Source: CAD feature listing. Evaluate the final solid. Frame: model axes, mm. A direction names the side the tool comes from. Coordinates: 2 decimals unless noted, no trailing zeros. Order: outer loops, then holes, each group sorted by start corner. A loop starts at its lowest first (then second) coordinate and runs counter-clockwise, first axis right, second up.
Item 1: Section A-A on x = 0. Return the cut outline in (y, z).
Item 2: Section B-B on z = -10.26. Return the cut outline in (x, y).
Item 3: Reachability of faces 5 (the flat face through (17, -6, -16)), 6 (the flat face through (-1, -6, -18)) from +Z, -Z, +X, -X, +Y, -Y: full face, straight path, thin tool, end or side. Return the list, or none.
Item 4: Section D-D on z = -2.75. Return the cut outline in (x, y).
Item 5: Contact query for flat-ended pins moving along their axis: P1, Ø4, axis at x = -23, y = -5.5, coming from the +Z side; P2, Ø8, axis at x = -25.5, z = -6.5, coming from the -Y side. Output: stop coordinate, or through.
Item 6: Section C-C on y = -4. Return the cut outline in (x, z).
Item 7: Ray query, line 1 (X direction, y = -1.05, z = -10.26); line 2 (X direction, y = -2.75, z = -0.75); line 3 (Z direction, x = -25.5, y = -6.25). Return the intervals inside material, ascending.
Item 8: Mould query, pull axis Z, two halves, no side actions, for faces 1 (the cylindrical face through (0.11, -0.986, -12.758)), 2 (the cylindrical face through (-16.52, -0.99, -10.59)), 3 (the flat face through (46, -5, -9)), 4 (the cylindrical face through (-0.644, -0.713, -17.248)). Classes: released by +Z, released by -Z, zero draft, split by the parting line, or undercut.
from build123d import *

# Parameters (mm, degrees)
SKETCH1_W                    = 92
SKETCH1_H                    = 18
BASE_FLANGE1_DEPTH           = 2
SKETCH11_R                   = 2.5
CUT_EXTRUDE1_DEPTH           = 2
EDGE_FLANGE1_STRIP_W         = 9
EDGE_FLANGE1_STRIP_H         = 2
EDGE_FLANGE1_STRIP_CUT_DEPTH = 92
EDGE_FLANGE1_DEPTH           = 92
BOSS_EXTRUDE2_DEPTH          = 2
LPATTERN1_COUNT              = 2
LPATTERN1_PITCH              = 35.5


# Sheet-metal steps are written as plain solids
with BuildPart() as part:
    # Sketch1 → Base-Flange1 (new body)
    with BuildSketch(Plane(origin=(0, 0, 0), x_dir=(1, 0, 0), z_dir=(0, 1, 0))):
        with Locations((0, 9)):
            Rectangle(SKETCH1_W, SKETCH1_H)
    extrude(amount=-BASE_FLANGE1_DEPTH)

    # Sketch11 → Cut-Extrude1 (cut)
    with BuildSketch(Plane(origin=(0, 0, 0), x_dir=(1, 0, 0), z_dir=(0, 1, 0))):
        with Locations(Location((0, 10.26, 0), (0, 0, 270))):
            Circle(SKETCH11_R)
        with Locations(Location((-19, 10.26, 0), (0, 0, 270))):
            Circle(SKETCH11_R)
    extrude(amount=-CUT_EXTRUDE1_DEPTH, mode=Mode.SUBTRACT)

    # Edge-Flange1 strip (across the edge) → Edge-Flange1 strip cut (cut)
    with BuildSketch(Plane(origin=(-46, -2, -18), x_dir=(0, 0, 1), z_dir=(1, 0, 0))):
        with Locations((-2, -1)):
            Rectangle(EDGE_FLANGE1_STRIP_W, EDGE_FLANGE1_STRIP_H)
    extrude(amount=EDGE_FLANGE1_STRIP_CUT_DEPTH, mode=Mode.SUBTRACT)

    # Edge-Flange1 section (across the edge) → Edge-Flange1 (add)
    with BuildSketch(Plane(origin=(-46, -2, -18), x_dir=(0, 0, 1), z_dir=(1, 0, 0))):
        with BuildLine():
            Line((0, 0.5), (0, 8))
            Line((0, 8), (2, 8))
            Line((2, 8), (2, 0.5))
            ThreePointArc((2, 0.5), (2.146446609, 0.146446609), (2.5, 0))
            Line((2.5, 0), (2.5, -2))
            ThreePointArc((2.5, -2), (0.732233047, -1.267766953), (0, 0.5))
        make_face()
    extrude(amount=EDGE_FLANGE1_DEPTH)

    # Sketch18 → Boss-Extrude2 (add)
    with BuildSketch(Plane.ZY.offset(46)):
        with BuildLine():
            Line((0, -2), (-15.5, -2))
            ThreePointArc((-15.5, -2), (-15.853553391, -2.146446609), (-16, -2.5))
            Line((-16, -2.5), (-16, -10))
            Line((-16, -10), (0, -10))
            Line((0, -10), (0, -2))
        make_face()
    boss_extrude2 = extrude(amount=-BOSS_EXTRUDE2_DEPTH)

    # LPattern1: Boss-Extrude2 ×2
    with Locations(*[(i * LPATTERN1_PITCH, 0, 0) for i in range(1, LPATTERN1_COUNT)]):
        add(boss_extrude2)

    # Mirror2: Boss-Extrude2 across plane
    add(boss_extrude2.mirror(Plane(origin=(0, 0, 0), x_dir=(0, 0, 1), z_dir=(1, 0, 0))))


solid = part.part
Answer list:
1. outline: (-10, -18) - (-2.5, -18) arc R2.5 ccw to (0, -15.5) - (0, -12.76) - (-2, -12.76) - (-2, -15.5) arc R0.5 cw to (-2.5, -16) - (-10, -16) - close; (-2, -7.76) - (0, -7.76) - (0, 0) - (-2, 0) - close
2. outline: (-46, -10) - (-44, -10) - (-44, -2) - (-21.5, -2) - (-21.5, 0) - (-46, 0) - close; (-16.5, -2) - (-10.5, -2) - (-10.5, -10) - (-8.5, -10) - (-8.5, -2) - (-2.5, -2) - (-2.5, 0) - (-16.5, 0) - close; (2.5, -2) - (44, -2) - (44, -10) - (46, -10) - (46, 0) - (2.5, 0) - close
3. face 5: +Z, -Y
3. face 6: -Z, +X, -X, +Y, -Y
4. outline: (-46, -10) - (-44, -10) - (-44, -2) - (-10.5, -2) - (-10.5, -10) - (-8.5, -10) - (-8.5, -2) - (44, -2) - (44, -10) - (46, -10) - (46, 0) - (-46, 0) - close
5. P1: stops at z = -16
5. P2: stops at y = -2
6. outline: (-46, -18) - (46, -18) - (46, 0) - (44, 0) - (44, -16) - (-8.5, -16) - (-8.5, 0) - (-10.5, 0) - (-10.5, -16) - (-44, -16) - (-44, 0) - (-46, 0) - close
7. line 1: x = -46 to -21.5, -16.5 to -2.5, 2.5 to 46
7. line 2: x = -46 to -44, -10.5 to -8.5, 44 to 46
7. line 3: z = -18 to -16
8. face 1: undercut
8. face 2: undercut
8. face 3: zero draft
8. face 4: released by -Z
